Design review of the part built by this model. Coordinates are the model's own, in mm. Face numbers are marked on the shaded views. A direction names the side the tool comes from. Coordinates: 2 decimals unless noted, no trailing zeros. Loops run counter-clockwise (first coordinate to the right, second up) from the corner with the lowest first, then second, coordinate; pieces in that order, holes last.
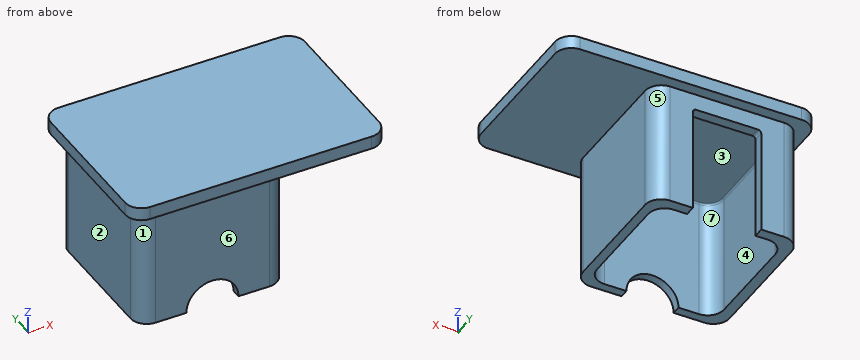
from build123d import *

# Parameters (mm, degrees)
F1_W      = 45
F1_H      = 45
F2_DEPTH  = 38
F0_W      = 39
F0_H      = 39
F3_DEPTH  = 37
F4_R      = 5
F5_R      = 0.5
F6_R      = 5
F7_R      = 8
F8_DEPTH  = 45.001
F9_W      = 52
F9_H      = 52
F10_DEPTH = 4
F11_R     = 5
F13_DEPTH = 11.9
F14_R     = 1
F16_W     = 31
F16_H     = 52
F17_DEPTH = 4
F18_R     = 5


with BuildPart() as f2:
    # F1 (on Top) → F2 (new body)
    with BuildSketch(Plane.XY):
        with Locations((32.002782, -21.252214)):
            Rectangle(F1_W, F1_H)
    extrude(amount=F2_DEPTH)

    # F0 (on Top) → F3 (cut)
    with BuildSketch(Plane.XY):
        with Locations((32.252782, -21.502214)):
            Rectangle(F0_W, F0_H)
    extrude(amount=F3_DEPTH, mode=Mode.SUBTRACT)

    # F4
    f4_edges = [f2.edges().sort_by_distance(p)[0] for p in [
        (12.752782, -41.002214, 18.5),
        (51.752782, -41.002214, 18.5),
        (51.752782, -2.002214, 18.5),
        (12.752782, -2.002214, 18.5),
    ]]
    fillet(f4_edges, radius=F4_R)

    # F5
    f5_edges = [f2.edges().sort_by_distance(p)[0] for p in [
        (51.752782, -21.502214, 37),
    ]]
    fillet(f5_edges, radius=F5_R)

    # F6
    f6_edges = [f2.edges().sort_by_distance(p)[0] for p in [
        (54.502782, 1.247786, 19),
        (54.502782, -43.752214, 19),
        (9.502782, -43.752214, 19),
        (9.502782, 1.247786, 19),
    ]]
    fillet(f6_edges, radius=F6_R)

    # F7 (on face) → F8 (cut, through all)
    with BuildSketch(Plane(origin=(0, 1.247786, 0), x_dir=(-1, 0, 0), z_dir=(0, 1, 0))):
        with Locations((-32.002782, 0)):
            Circle(F7_R)
    extrude(amount=-F8_DEPTH, mode=Mode.SUBTRACT)

    # F9 (on face) → F10 (join)
    with BuildSketch(Plane.XY.offset(38)):
        with Locations((32.002782, -21.252214)):
            Rectangle(F9_W, F9_H)
    extrude(amount=F10_DEPTH)

    # F11
    f11_edges = [f2.edges().sort_by_distance(p)[0] for p in [
        (6.002782, 4.747786, 40),
        (58.002782, 4.747786, 40),
        (58.002782, -47.252214, 40),
        (6.002782, -47.252214, 40),
    ]]
    fillet(f11_edges, radius=F11_R)

    # F12 (on face) → F13 (cut)
    with BuildSketch(Plane(origin=(0, 1.247786, 0), x_dir=(-1, 0, 0), z_dir=(0, 1, 0))):
        with BuildLine():
            Line((-42.502782, 33), (-42.502782, 0))
            Line((-42.502782, 0), (-40.002782, 0))
            ThreePointArc((-40.002782, 0), (-32.002782, 8), (-24.002782, 0))
            Line((-24.002782, 0), (-21.502782, 0))
            Line((-21.502782, 0), (-21.502782, 33))
            Line((-21.502782, 33), (-42.502782, 33))
        make_face()
    extrude(amount=-F13_DEPTH, mode=Mode.SUBTRACT)

    # F14
    f14_edges = [f2.edges().sort_by_distance(p)[0] for p in [
        (21.502782, -0.377214, 33),
        (42.502782, -0.377214, 33),
    ]]
    fillet(f14_edges, radius=F14_R)

    # F16 (on face) → F17 (join)
    with BuildSketch(Plane.XY.offset(42)):
        with Locations((68.502782, -21.252214)):
            Rectangle(F16_W, F16_H)
    extrude(amount=-F17_DEPTH)

    # F18
    f18_edges = [f2.edges().sort_by_distance(p)[0] for p in [
        (84.002782, 4.747786, 40),
        (84.002782, -47.252214, 40),
    ]]
    fillet(f18_edges, radius=F18_R)


solid = f2.part
Q1. Take a section at C-C, the plane z = 23.5. Write out the cut boundary in (x, y).
Q2. Take a section at A-A, the plane y = -13. Write out the cut boundary in (x, z), then the cut area to 3 significant figures.
Q3. Take a section at D-D, the plane x = 67. Write out the cut boundary in (y, z).
Q4. Take a section at B-B, the plane z = 7. Write out the cut boundary in (x, y), then the cut area to 3 significant figures.
Q5. For line 1 (Y direction, x = 45, z = 14); line 2 (X direction, y = -22, z = 33.5); line 3 (X direction, y = -42, z = 6.5), list the stretches that pass through material, from the lowest coordinate up.
Q6. Machinability: for the marked faces 5, 6 and 7, which of the approach directions +Z, -Z, +X, -X, +Y, -Y give a long, thin tool a straight path to every point of the face, cutting with its end or side? Answer none if there is none.
Q7. Clearance check with flat-ended pins moving along their axes: pin 1 Ø5 at (x, z) = (38.5, 16) entering from +Y; pin 2 Ø1.5 at (y, z) = (-38, 26) entering from -X; pin 3 Ø8.5 at (y, z) = (-19, 10.5) entering from +X. State where each tip first meets the part, or that it passes through.
Q8. The part is to be moulded in two halves that separate along Y. For the marked faces 1, 2, 3 and 4, say which applies: pulls with the +Y half, pulls with the -Y half, needs draft (parallel to the pull), parting line crosses it, or undercut.
Entries:
1. outline: (9.5, -38.75) arc R5 ccw to (14.5, -43.75) - (49.5, -43.75) arc R5 ccw to (54.5, -38.75) - (54.5, -3.75) arc R5 ccw to (49.5, 1.25) - (42.5, 1.25) - (42.5, -2) - (46.75, -2) arc R5 cw to (51.75, -7) - (51.75, -36) arc R5 cw to (46.75, -41) - (17.75, -41) arc R5 cw to (12.75, -36) - (12.75, -7) arc R5 cw to (17.75, -2) - (21.5, -2) - (21.5, 1.25) - (14.5, 1.25) arc R5 ccw to (9.5, -3.75) - close
2. outline: (6, 38) - (9.5, 38) - (9.5, 0) - (12.75, 0) - (12.75, 36.5) arc R0.5 cw to (13.25, 37) - (51.25, 37) arc R0.5 cw to (51.75, 36.5) - (51.75, 0) - (54.5, 0) - (54.5, 38) - (84, 38) - (84, 42) - (6, 42) - close
2. area: 579 mm2
3. outline: (-47.25, 38) - (4.75, 38) - (4.75, 42) - (-47.25, 42) - close
4. outline: (9.5, -38.75) arc R5 ccw to (14.5, -43.75) - (28.13, -43.75) - (28.13, -41) - (17.75, -41) arc R5 cw to (12.75, -36) - (12.75, -7) arc R5 cw to (17.75, -2) - (21.5, -2) - (21.5, 1.25) - (14.5, 1.25) arc R5 ccw to (9.5, -3.75) - close; (35.88, -43.75) - (49.5, -43.75) arc R5 ccw to (54.5, -38.75) - (54.5, -3.75) arc R5 ccw to (49.5, 1.25) - (42.5, 1.25) - (42.5, -2) - (46.75, -2) arc R5 cw to (51.75, -7) - (51.75, -36) arc R5 cw to (46.75, -41) - (35.88, -41) - close
4. area: 414 mm2
5. line 1: y = -43.75 to -41, -2 to 1.25
5. line 2: x = 9.5 to 12.75, 51.75 to 54.5
5. line 3: x = 10.7 to 27.34, 36.67 to 53.3
6. face 5: -Z, +X, +Y
6. face 6: -Z, +X, -X, -Y
6. face 7: -Z
7. pin 1: stops at y = -41
7. pin 2: stops at x = 9.5
7. pin 3: stops at x = 54.5
8. face 1: pulls with the -Y half
8. face 2: needs draft
8. face 3: undercut
8. face 4: undercut
